```python
from build123d import *

# Parameters (mm, degrees)
SKETCH_2_R      = 2
EXTRUDE_1_DEPTH = 2.5


with BuildPart() as part:
    # 草圖2 → 填料-伸長1 (new, symmetric)
    with BuildSketch(Plane.XY):
        with BuildLine():
            Line((27.034153101, 30.363667163), (67.906299219, 3.336501724))
            ThreePointArc((67.906299219, 3.336501724), (69.530535661, -1.151953364), (65.7, -4))
            Line((65.7, -4), (52.175653003, 2.831217066))
            ThreePointArc((52.175653003, 2.831217066), (30.231729467, 7.633890773), (8.700316547, 1.230788983))
            Line((8.700316547, 1.230788983), (0, -4))
            ThreePointArc((0, -4), (-3.662248796, -1.608705616), (-2.945740102, 2.706033121))
            Line((-2.945740102, 2.706033121), (21.882113779, 29.733198559))
            ThreePointArc((21.882113779, 29.733198559), (24.341987779, 30.997547553), (27.034153101, 30.363667163))
        make_face()
        Circle(SKETCH_2_R, mode=Mode.SUBTRACT)
        with Locations((24.827853881, 27.027165439)):
            Circle(SKETCH_2_R, mode=Mode.SUBTRACT)
    extrude(amount=EXTRUDE_1_DEPTH, both=True)


solid = part.part
```
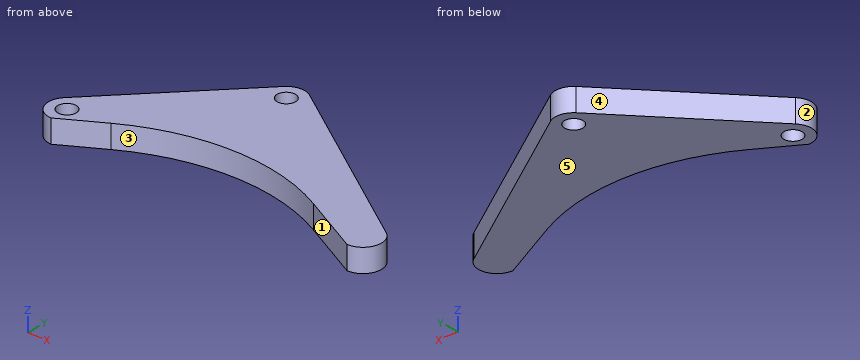
Model file for the job. Use its own axes, mm. Face numbers are marked on the shaded views. A direction names the side the tool comes from. Give positions to 0.01 mm unless a question says otherwise; leave off trailing zeros. Loops run counter-clockwise (first coordinate to the right, second up) from the corner with the lowest first, then second, coordinate; pieces in that order, holes last. Notation, with made-up numbers: M -28,86 L -8,86 A23 cw -8,109 Z; hole C 80,24.25 d10. An arc over 180 degrees is marked long. Use one line per item in the form item = value.
Item 1: Drill centre lines: L1, parallel to Y at x = 0, z = 0.1; L2, parallel to X at y = 28, z = -1.25; L3, parallel to X at y = 27, z = -1.9. Where is each one in solid material? Low to high.
Filled in:
L1 = -4 to -2, 2 to 5.91
L2 = 20.29 to 23.08, 26.58 to 30.61
L3 = 19.37 to 22.83, 26.83 to 32.12
Item 2: Slice it at B-B on y = 0. List the corners of the cut face in (x, z).
Filled in:
outline = M -4,-2.5 L -2,-2.5 L -2,2.5 L -4,2.5 Z; M 2,-2.5 L 6.65,-2.5 L 6.65,2.5 L 2,2.5 Z; M 57.78,-2.5 L 69.7,-2.5 L 69.7,2.5 L 57.78,2.5 Z
Item 3: Slice it at C-C on z = -1.05. List the corners of the cut face in (x, y).
Filled in:
outline = M -2.95,2.71 A4 ccw 0,-4 L 8.7,1.23 A45 cw 52.18,2.83 L 65.7,-4 A4 ccw 67.91,3.34 L 27.03,30.36 A4 ccw 21.88,29.73 Z; hole C 0,0 d4; hole C 24.83,27.03 d4
Item 4: Flat gauge pins, fed straight in: pin 1 Ø3 at (x, y) = (24.83, 27.03) entering from -Z; pin 2 Ø2 at (y, z) = (8, -0.5) entering from +X. Where does each tip first touch, or does it go through?
Filled in:
pin_1 = through
pin_2 = 62.37
Item 5: Two-plate mould, pull along X, no slides. Class the marked faces 3, 4 and 5: released by +X, released by -X, zero draft, split by the parting line, or undercut.
Filled in:
face_3 = undercut
face_4 = released by -X
face_5 = zero draft
Item 6: Slice it at A-A on x = 25. List the corners of the cut face in (y, z).
Filled in:
outline = M 7.13,-2.5 L 25.03,-2.5 L 25.03,2.5 L 7.13,2.5 Z; M 29.02,-2.5 L 31.02,-2.5 L 31.02,2.5 L 29.02,2.5 Z
Item 7: Which spindle directions (+Z, -Z, +X, -X, +Y, -Y) get a long thin tool onto all of the face, cutting with end or side? Do the marked faces 1 and 2. Say none if no direction does.
Filled in:
face_1 = +Z, -Z, -Y
face_2 = +Z, -Z, -X
Item 8: Slice it at D-D on x = 63. List the corners of the cut face in (y, z), and give its area (3 significant figures).
Filled in:
outline = M -2.64,-2.5 L 6.58,-2.5 L 6.58,2.5 L -2.64,2.5 Z
area = 46.1 mm^2
